Model file for the job. Use its own axes, mm. Coordinates: 2 decimals unless noted, no trailing zeros. Write each loop counter-clockwise with the first axis right and the second up, starting at its lowest first coordinate (ties: lowest second). Pieces come first, ordered by that corner, then holes. Notation, with made-up numbers: M -14.75,-31 L 13.25,-31 A22 cw 13.25,-18 Z; hole C -11,37.5 d8. An arc over 180 degrees is marked long. Use CSV: the item, a comma, the result in double quotes. Start each with the question number.
Autodesk Inventor part; units mm, degrees
ref_plane "YZ Plane" through (0, 0, 0) normal (1, 0, 0) x (0, 1, 0)
ref_plane "XZ Plane" through (0, 0, 0) normal (0, 1, 0) x (-1, 0, 0)
ref_plane "XY Plane" through (0, 0, 0) normal (0, 0, 1) x (1, 0, 0)
sketch "Sketch1" plane through (0, 0, 0) normal (0, 1, 0) x (-1, 0, 0)
  line L0 (1.7321, -13.5333) -> (-1.7321, -13.5333)
  line L1 (-1.7321, -13.5333) -> (-12.5862, 5.2667)
  line L2 (-12.5862, 5.2667) -> (-10.8542, 8.2667)
  line L3 (-10.8542, 8.2667) -> (10.8542, 8.2667)
  line L4 (10.8542, 8.2667) -> (12.5862, 5.2667)
  line L5 (12.5862, 5.2667) -> (1.7321, -13.5333)
  circle A0 centre (0, 0) radius 8.2667 construction
  point P0 (0, -16.5333)
  dimension "d0" = 21.8
  dimension "d1" = 3.4641
  dimension "d4" = 24.8
extrude "Extrusion1" add sketch "Sketch1" along normal mid plane 1.75
equation "\"d0\" = TriangleTrimmed"
properties part number "CommandToken_Single" material "Paper"
1) Band-saw the part on C-C on z = 1.25. List the corners of the cut face in (x, y) (3 decimals), then the cut area to 3 significant figures.
2) Two-plate mould, pull along Z, no slides. Class faces 1 (the face through (7.083, -0.012, -4.265)), 2 (the face through (0, 0.875, 0)), 3 (the face through (11.73, -0.01, 6.75)): pulls with the +Z half, pulls with the -Z half, needs draft (parallel to the pull), parting line crosses it, or undercut.
3) Band-saw the part on B-B on x = 4.5. List the corners of the cut face in (y, z) (3 decimals), then the cut area to 3 significant figures.
4) Wall check: L1, parallel to X at y = 0.75, z = 6.5; L2, parallel to X at y = -0.5, z = -0.75; L3, parallel to Z at x = -8.25, y = -0.5. Give the ranges that are in metal, low to high. Write a range as [from, to].
5) Band-saw the part on A-A on y = 0. List the corners of the cut face in (x, z), then the cut area to 3 significant figures.
Findings below:
1,outline,"M -10.267,-0.875 L 10.267,-0.875 L 10.267,0.875 L -10.267,0.875 Z"
1,area,"35.9 mm2"
2,face 1,"pulls with the -Z half"
2,face 2,"needs draft"
2,face 3,"pulls with the +Z half"
3,outline,"M -0.875,-8.739 L 0.875,-8.739 L 0.875,8.267 L -0.875,8.267 Z"
3,area,"29.8 mm2"
4,L1,"x = [-11.87, 11.87]"
4,L2,"x = [-9.11, 9.11]"
4,L3,"z = [-2.24, 8.27]"
5,outline,"M -12.59,5.27 L -1.73,-13.53 L 1.73,-13.53 L 12.59,5.27 L 10.85,8.27 L -10.85,8.27 Z"
5,area,"340 mm2"
